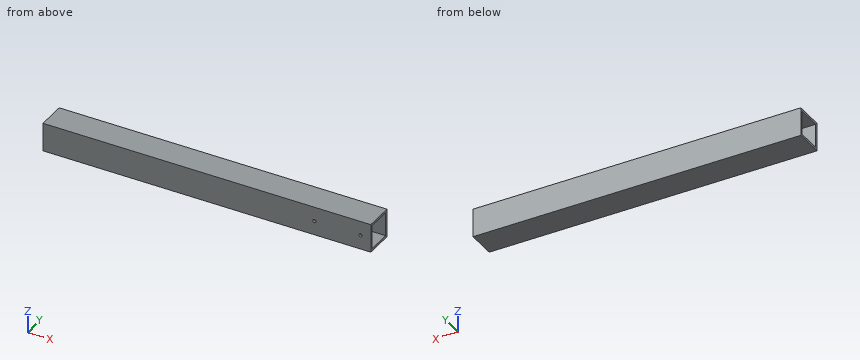
from build123d import *

# Parameters (mm, degrees)
F0_W     = 76.2
F0_H     = 76.2
F0_W_2   = 63.5
F0_H_2   = 63.5
F1_DEPTH = 876.3
F4_D     = 8.8
F4_DEPTH = 29.15
F4_TIP   = 2.6437867237


with BuildPart() as f1:
    # F0 (on Right) → F1 (new body)
    with BuildSketch(Plane.YZ):
        with Locations((1.4744321764, 0.1075561106)):
            Rectangle(F0_W, F0_H)
        with Locations((1.4744321764, 0.1075561106)):
            Rectangle(F0_W_2, F0_H_2, mode=Mode.SUBTRACT)
    extrude(amount=F1_DEPTH)

    # F4
    with Locations(Plane.XZ.offset(36.6255678236)):
        with Locations((848.8616235588, 0), (725.4748, 0)):
            Hole(F4_D / 2, depth=F4_DEPTH)
            with Locations((0, 0, -(F4_DEPTH + F4_TIP / 2))):  # 118° drill point
                Cone(0, F4_D / 2, F4_TIP, mode=Mode.SUBTRACT)


solid = f1.part
CAD build for the part. Positions are in the model's coordinates, mm. Coordinates: 2 decimals unless noted, no trailing zeros. Order: outer loops, then holes, each group sorted by start corner. A loop starts at its lowest first (then second) coordinate and runs counter-clockwise, first axis right, second up.
Item 1: Pin check, flat tips, straight feed: pin 1 Ø12 at (y, z) = (3, 21) entering from -X; pin 2 Ø10 at (y, z) = (28.5, 9.5) entering from +X. Stop position of each tip, or through.
Check sheet entries:
pin 1: passes through
pin 2: stops at x = 876.3
Item 2: Band-saw the part on A-A on y = 18.5. List the corners of the cut face in (x, z).
Check sheet entries:
outline: (0, -37.99) - (876.3, -37.99) - (876.3, -31.64) - (0, -31.64) - close; (0, 31.86) - (876.3, 31.86) - (876.3, 38.21) - (0, 38.21) - close
Item 3: Band-saw the part on B-B on x = 87.5. List the corners of the cut face in (y, z), plus the area to 3 significant figures.
Check sheet entries:
outline: (-36.63, -37.99) - (39.57, -37.99) - (39.57, 38.21) - (-36.63, 38.21) - close; hole (-30.28, -31.64) - (33.22, -31.64) - (33.22, 31.86) - (-30.28, 31.86) - close
area: 1,770 mm2
Item 4: Drill centre lines: L1, parallel to Y at x = 711, z = 27.5; L2, parallel to Z at x = 338.5, y = -7. Where is each one in solid material? Low to high.
Check sheet entries:
L1: y = -36.63 to -30.28, 33.22 to 39.57
L2: z = -37.99 to -31.64, 31.86 to 38.21
